Can you work these out from the model? Positions are in its coordinate system, mm. A direction names the side the tool comes from. Round coordinates to 2 decimals unless told otherwise and drop trailing zeros. Order: outer loops, then holes, each group sorted by start corner. A loop starts at its lowest first (then second) coordinate and runs counter-clockwise, first axis right, second up. Notation, with made-up numbers: M 83.5,6 L 137.5,6 A22 ccw 137.5,31 Z; hole C 34,58 d11. An arc over 180 degrees is marked long. Answer as CSV lines item,"result". Start each with the question number.
from build123d import *

# Parameters (mm, degrees)
SKETCH1_W           = 44.45
SKETCH1_H           = 30.48
BOSS_EXTRUDE1_DEPTH = 7.62
SKETCH2_R           = 1.0795
BOSS_EXTRUDE2_DEPTH = 2.54
SKETCH3_R           = 7.9375
CUT_EXTRUDE1_DEPTH  = 5.08
SKETCH4_W           = 15.24
SKETCH4_H           = 30.48
CUT_EXTRUDE2_DEPTH  = 6.35
SKETCH5_W           = 4.445
SKETCH5_H           = 30.48
CUT_EXTRUDE3_DEPTH  = 4.318
BOSS_EXTRUDE3_DEPTH = 2.032


with BuildPart() as part:
    # Sketch1 → Boss-Extrude1 (new body)
    with BuildSketch(Plane.XY):
        with Locations((22.225, 15.24)):
            Rectangle(SKETCH1_W, SKETCH1_H)
    extrude(amount=BOSS_EXTRUDE1_DEPTH)

    # Sketch2 → Boss-Extrude2 (add)
    with BuildSketch(Plane.XY.offset(7.62)):
        with Locations(Location((6.35, 24.765, 0), (0, 0, 180))):
            Circle(SKETCH2_R)
        with Locations(Location((6.35, 5.715, 0), (0, 0, 180))):
            Circle(SKETCH2_R)
        with Locations(Location((11.43, 24.765, 0), (0, 0, 180))):
            Circle(SKETCH2_R)
        with Locations(Location((19.7513587, 27.686, 0), (0, 0, 180))):
            Circle(SKETCH2_R)
        with Locations(Location((19.7513587, 2.794, 0), (0, 0, 180))):
            Circle(SKETCH2_R)
    extrude(amount=BOSS_EXTRUDE2_DEPTH)

    # Sketch3 → Cut-Extrude1 (cut)
    with BuildSketch(Plane.XY.offset(7.62)):
        with Locations((0, 15.24)):
            Circle(SKETCH3_R)
    extrude(amount=-CUT_EXTRUDE1_DEPTH, mode=Mode.SUBTRACT)

    # Sketch4 → Cut-Extrude2 (cut)
    with BuildSketch(Plane.XY.offset(7.62)):
        with Locations((36.83, 15.24)):
            Rectangle(SKETCH4_W, SKETCH4_H)
    extrude(amount=-CUT_EXTRUDE2_DEPTH, mode=Mode.SUBTRACT)

    # Sketch5 → Cut-Extrude3 (cut)
    with BuildSketch(Plane.XY.offset(7.62)):
        with Locations((26.9875, 15.24)):
            Rectangle(SKETCH5_W, SKETCH5_H)
    extrude(amount=-CUT_EXTRUDE3_DEPTH, mode=Mode.SUBTRACT)

    # Sketch6 → Boss-Extrude3 (add)
    with BuildSketch(Plane.XY.offset(1.27)):
        Polygon((29.21, 0), (29.21, 1.93778588), (32.678761959, 1.93778588), (32.678761959, 3.133507731), (37.686930292, 3.133507731), (37.686930292, 8.402137785), (32.658263267, 8.402137785), (32.658263267, 9.590598202), (29.21, 9.590598202), (29.21, 10.097072894), (32.658263267, 10.097072894), (32.658263267, 11.322249124), (41.237467305, 11.322249124), (41.237467305, 19.177308186), (32.703717585, 19.177308186), (32.703717585, 20.417489762), (29.21, 20.417489762), (29.21, 20.9492523), (32.703717585, 20.9492523), (32.703717585, 22.079298556), (37.771400605, 22.079298556), (37.771400605, 27.473279734), (32.702551474, 27.473279734), (32.702551474, 28.622642458), (29.21, 28.622642458), (29.21, 30.48), (44.45, 30.48), (44.45, 0), align=None)
    extrude(amount=BOSS_EXTRUDE3_DEPTH)


solid = part.part
(1) If I drill on line 1 along X through (y, z) = (7, 2.5); line 2 along X through (y, z) = (14.5, 2); line 3 along X through (y, z) = (3.5, 5.5) (3 decimals), over which ranges is the centre line in solid material (lowest first)?
(2) For faces 5 (the flat face through (18, 0, 3)), 6 (the flat face through (37.687, 6, 2)), which set-ups out of +Z, -Z, +X, -X, +Y, -Y let a thin tool reach every point of the face, with its end or its side?
(3) I want a section at D-D on z = 4.5. Write out the boundary of the cut face in (x, y) (1 decimal).
(4) I'm going to push flat-ended pins straight in: P1, Ø3, axis at x = 36, y = 17.5, coming from the +Z side; P2, Ø2, axis at x = 10.5, y = 6.5, coming from the +Z side; P3, Ø2.5, axis at x = 3, y = 18.5, coming from the +Z side. Where does each tip first touch, or does it pass through?
(5) I want a section at A-A on x = 37. Write out the boundary of the cut face in (y, z).
(6) If we mould it in two halves opening along X, with no side actions, what happens to faces 1 (the flat face through (44.45, 15, 2)), 2 (the flat face through (29.21, 15, 2)), 3 (the flat face through (0, 15, 2)), 4 (the flat face through (6, 6, 10.16))? For each: +X half, -X half, draft (parallel to the pull), parting line (faces both ways), or undercut.
(7) I want a section at C-C on z = 8.75. Count the separate pieces of the cut face and the enclosed holes in it, and give its area (3 significant figures).
From the geometry:
1,line 1,"0 to 29.21, 37.69 to 44.45"
1,line 2,"0 to 29.21, 41.24 to 44.45"
1,line 3,"0 to 24.765"
2,face 5,"+Z, -Z, +X, -X, -Y"
2,face 6,"+Z"
3,outline,"M 0,0 L 24.8,0 L 24.8,30.5 L 0,30.5 L 0,23.2 A7.9 cw 0,7.3 Z"
4,P1,"z = 1.27"
4,P2,"z = 7.62"
4,P3,"z = 2.54"
5,outline,"M 0,0 L 30.48,0 L 30.48,3.3 L 27.47,3.3 L 27.47,1.27 L 22.08,1.27 L 22.08,3.3 L 19.18,3.3 L 19.18,1.27 L 11.32,1.27 L 11.32,3.3 L 8.4,3.3 L 8.4,1.27 L 3.13,1.27 L 3.13,3.3 L 0,3.3 Z"
6,face 1,"+X half"
6,face 2,"undercut"
6,face 3,"-X half"
6,face 4,"draft"
7,separate pieces,"5"
7,enclosed holes,"0"
7,area,"18.3 mm²"
